```python
from build123d import *

# Parameters (mm, degrees)
BOSS_EXTRUDE1_DEPTH = 19.05
SKETCH1_4_R         = 1.5875
CUT_EXTRUDE2_DEPTH  = 9.525
SKETCH2_R           = 1.5875
CUT_EXTRUDE3_DEPTH  = 21.83438774


with BuildPart() as part:
    # Sketch1 → Boss-Extrude1 (new body)
    with BuildSketch(Plane(origin=(0, 0, 0), x_dir=(1, 0, 0), z_dir=(0, 1, 0))):
        with BuildLine():
            Line((-7.9375, 0), (0, 0))
            ThreePointArc((0, 0), (-0.502011579, 0.081465264), (-0.9525, 0.3175))
            Line((-0.9525, 0.3175), (-7.9375, 0.3175))
            Line((-7.9375, 0.3175), (-7.9375, 0))
        make_face()
        with BuildLine():
            Line((0, 0), (0, 0.3175))
            Line((0, 0.3175), (-0.9525, 0.3175))
            ThreePointArc((-0.9525, 0.3175), (-0.502011579, 0.081465264), (0, 0))
        make_face()
        with BuildLine():
            Line((-0.9525, 0.3175), (0, 0.3175))
            Line((0, 0.3175), (0, 0))
            ThreePointArc((0, 0), (1.122532015, 0.464967985), (1.5875, 1.5875))
            ThreePointArc((1.5875, 1.5875), (-0.709951583, 3.007403166), (-0.9525, 0.3175))
        make_face()
    extrude(amount=BOSS_EXTRUDE1_DEPTH)

    # Sketch1_4 → Cut-Extrude2 (cut)
    with BuildSketch(Plane(origin=(0, 0, 0), x_dir=(1, 0, 0), z_dir=(0, 1, 0))):
        with Locations((0, 1.5875)):
            Circle(SKETCH1_4_R)
    extrude(amount=CUT_EXTRUDE2_DEPTH, mode=Mode.SUBTRACT)

    # Sketch2 → Cut-Extrude3 (cut, through all)
    with BuildSketch(Plane(origin=(0, 0, -0.3175), x_dir=(-1, 0, 0), z_dir=(0, 0, -1))):
        with Locations((4.7625, 15.08125)):
            Circle(SKETCH2_R)
        with Locations((4.7625, 3.96875)):
            Circle(SKETCH2_R)
    extrude(amount=-CUT_EXTRUDE3_DEPTH, mode=Mode.SUBTRACT)


solid = part.part
```
Source: CAD feature listing. Evaluate the final solid. Frame: model axes, mm. A direction names the side the tool comes from. Give positions to 0.01 mm unless a question says otherwise; leave off trailing zeros. Loops run counter-clockwise (first coordinate to the right, second up) from the corner with the lowest first, then second, coordinate; pieces in that order, holes last. Notation, with made-up numbers: (28.5, -6) - (66.5, -6) arc R35 cw to (66.5, 32) - close; hole circle Ø5 at (70, -39.5). An arc over 180 degrees is marked (long way). Use CSV: the item, a comma, the result in double quotes. Start each with the question number.
1. Ray query, L1, parallel to Y at x = -0.75, z = -2.35 (3 decimals); L2, parallel to Z at x = -4.75, y = 6.25; L3, parallel to X at y = 15, z = -1.65. Return the intervals inside material, ascending.
2. Section A-A (x = -4). Output: boundary loops of the cut face in (y, z), then the cut area to 3 significant figures.
3. Section D-D (x = -6). Output: boundary loops of the cut face in (y, z), then the cut area to 3 significant figures.
4. Pin query (flat end, axial travel): pin 1 (5 mm diameter, centred on x = -7, y = 7, fed in from +Z); pin 2 (4 mm diameter, centred on x = -4.76, y = 3.97, fed in from -Z). Return the tip coordinate at first contact, or that it passes through.
5. Reachability of faces 1 (the cylindrical face through (-0.718, 4.696, -0.172)), 2 (the flat face through (-1, 19.05, -1)) from +Z, -Z, +X, -X, +Y, -Y: full face, straight path, thin tool, end or side. Return the list, or none.
Response:
1,L1,"9.525 to 19.05"
1,L2,"-0.32 to 0"
1,L3,"-1.59 to 1.59"
2,outline,"(0, -0.32) - (2.58, -0.32) - (2.58, 0) - (0, 0) - close; (5.36, -0.32) - (13.69, -0.32) - (13.69, 0) - (5.36, 0) - close; (16.47, -0.32) - (19.05, -0.32) - (19.05, 0) - (16.47, 0) - close"
2,area,"4.28 mm²"
3,outline,"(0, -0.32) - (2.97, -0.32) - (2.97, 0) - (0, 0) - close; (4.96, -0.32) - (14.09, -0.32) - (14.09, 0) - (4.96, 0) - close; (16.08, -0.32) - (19.05, -0.32) - (19.05, 0) - (16.08, 0) - close"
3,area,"4.79 mm²"
4,pin 1,"z = 0"
4,pin 2,"z = -0.32"
5,face 1,"-Z, +X, -Y"
5,face 2,"+Z, -Z, +X, -X, +Y"
